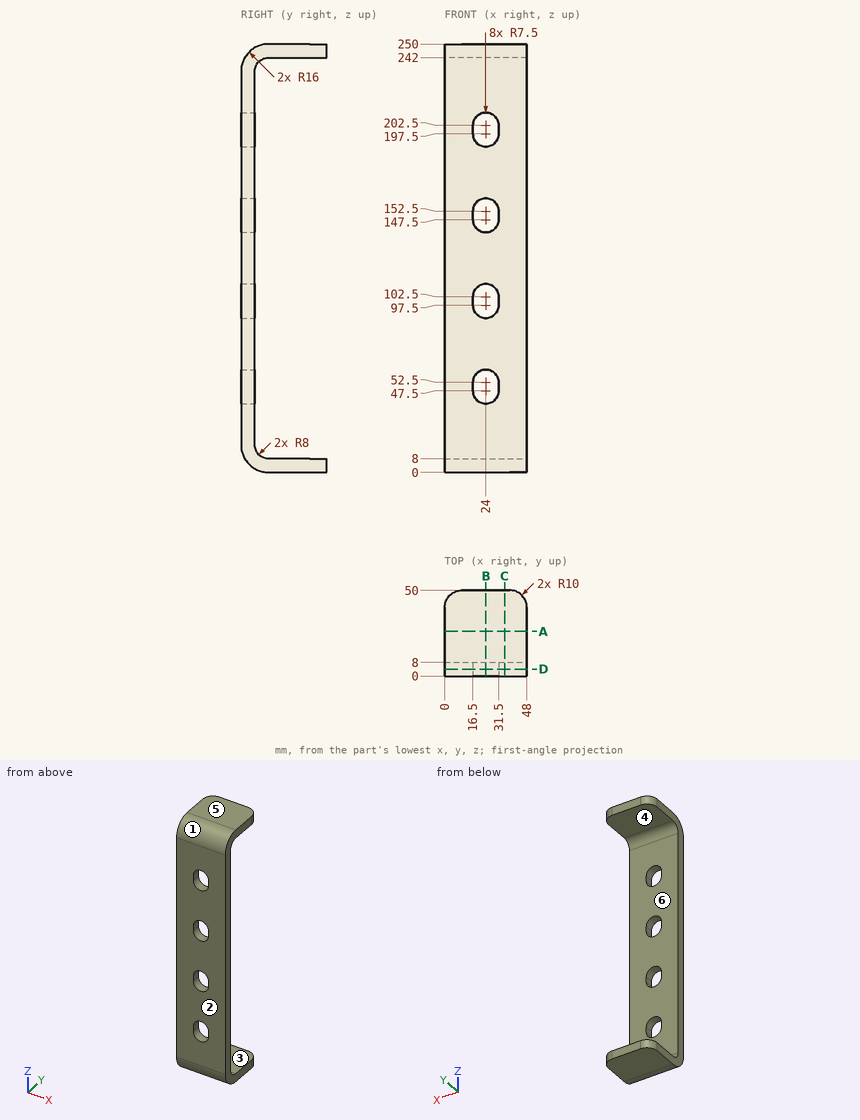
Geometry check sheet. Reference: drawing and pictorial views, mm from the part's lowest x, y, z. A direction names the side the tool comes from. Round coordinates to 2 decimals unless told otherwise and drop trailing zeros. Write each loop counter-clockwise with the first axis right and the second up, starting at its lowest first coordinate (ties: lowest second). Pieces come first, ordered by that corner, then holes.
Item 1: Go/stop test with flat-tipped pins: pin 1 Ø4 at (y, z) = (4, 51) entering from -X; pin 2 Ø8 at (x, y) = (41.5, 6.5) entering from +Z (3 decimals); pin 3 Ø8 at (x, z) = (24.5, 145) entering from +Y; pin 4 Ø10 at (x, z) = (18.5, 219) entering from +Y. Record where each tip stops, or that it passes through.
Determined:
pin 1: stops at x = 0
pin 2: stops at z = 249.025
pin 3: passes through
pin 4: stops at y = 8
Item 2: Mould release check, pull along Z, two halves, no side actions. Record for the marked faces 1, 2, 3 and 4: +Z half, -Z half, draft (parallel to the pull), parting line (faces both ways), or undercut.
Determined:
face 1: +Z half
face 2: draft
face 3: undercut
face 4: undercut
Item 3: Access from +Z, -Z, +X, -X, +Y, -Y to the whole of each face (thin tool, end or side, straight path). Record for the marked faces 5 and 6.
Determined:
face 5: +Z, +X, -X, +Y, -Y
face 6: +X, -X, +Y
Item 4: Section check D-D (y = 4). Record the boundary of the cut face in (x, z).
Determined:
outline: (0, 5.42) - (48, 5.42) - (48, 244.58) - (0, 244.58) - close; hole (16.5, 47.5) arc R7.5 ccw to (31.5, 47.5) - (31.5, 52.5) arc R7.5 ccw to (16.5, 52.5) - close; hole (16.5, 97.5) arc R7.5 ccw to (31.5, 97.5) - (31.5, 102.5) arc R7.5 ccw to (16.5, 102.5) - close; hole (16.5, 147.5) arc R7.5 ccw to (31.5, 147.5) - (31.5, 152.5) arc R7.5 ccw to (16.5, 152.5) - close; hole (16.5, 197.5) arc R7.5 ccw to (31.5, 197.5) - (31.5, 202.5) arc R7.5 ccw to (16.5, 202.5) - close
Item 5: Section check C-C (x = 35). Record the boundary of the cut face in (y, z).
Determined:
outline: (0, 16) arc R16 ccw to (16, 0) - (50, 0) - (50, 8) - (16, 8) arc R8 cw to (8, 16) - (8, 234) arc R8 cw to (16, 242) - (50, 242) - (50, 250) - (16, 250) arc R16 ccw to (0, 234) - close
Item 6: Section check B-B (x = 24). Record the boundary of the cut face in (y, z).
Determined:
outline: (0, 16) arc R16 ccw to (16, 0) - (50, 0) - (50, 8) - (16, 8) arc R8 cw to (8, 16) - (8, 40) - (0, 40) - close; (0, 60) - (8, 60) - (8, 90) - (0, 90) - close; (0, 110) - (8, 110) - (8, 140) - (0, 140) - close; (0, 160) - (8, 160) - (8, 190) - (0, 190) - close; (0, 210) - (8, 210) - (8, 234) arc R8 cw to (16, 242) - (50, 242) - (50, 250) - (16, 250) arc R16 ccw to (0, 234) - close
Item 7: Section check A-A (y = 26). Record the boundary of the cut face in (x, z), plus the area to 3 significant figures.
Determined:
outline: (0, 0) - (48, 0) - (48, 8) - (0, 8) - close; (0, 242) - (48, 242) - (48, 250) - (0, 250) - close
area: 768 mm2
Item 8: Material ranges on line 1 along Z through (x, y) = (7.5, 47); line 2 along X through (y, z) = (5.5, 99.5); line 3 along Y through (x, z) = (15.5, 57), recorded low to high.
Determined:
line 1: z = 0 to 8, 242 to 250
line 2: x = 0 to 16.5, 31.5 to 48
line 3: y = 0 to 8
